For this review, use the dimensioned drawing (mm, ordinates from the lowest corner) and the shaded views. A direction names the side the tool comes from. Round coordinates to 2 decimals unless told otherwise and drop trailing zeros. Loops run counter-clockwise (first coordinate to the right, second up) from the corner with the lowest first, then second, coordinate; pieces in that order, holes last. Notation, with made-up numbers: M -13.5,58 L 13.5,58 A30 ccw 13.5,90 Z; hole C 58.25,15.5 d5. An arc over 180 degrees is marked long. One line per item, written item: value. Start each with the question number.
Item 1: For line 1 along Y through (x, z) = (32.25, 12.5); line 2 along Y through (x, z) = (32, 3); line 3 along Y through (x, z) = (31, 14.25), list the stretches that pass through material, from the lowest coordinate up.
Item 2: We need section A-A (x = 38). Write out the cut boundary in (y, z).
Item 3: We need section B-B (y = 50). Write out the cut boundary in (x, z).
Item 4: Clearance check with flat-ended pins moving along their axes: pin 1 (1.5 mm diameter, centred on x = 30, z = 10.5, fed in from -Y); pin 2 (2.5 mm diameter, centred on y = 48.5, z = 12, fed in from +X). State where each tip first meets the part, or that it passes through.
Item 5: We need section C-C (x = 22). Write out the cut boundary in (y, z), then the cut area to 3 significant figures.
Item 6: For the marked faces 5 and 6, list the 3-axis set-ups (+Z, -Z, +X, -X, +Y, -Y) from which the entire face can be reached by the end or side of a thin tool; tool diameter is ignored.
Item 7: We need section D-D (z = 12.5). Write out the cut boundary in (x, y), then the cut area to 3 significant figures.
Item 8: Mouldability with a two-part tool opening along Z and no side actions: class the marked faces 1, 2, 3 and 4 as released by +Z, released by -Z, zero draft, split by the parting line, or undercut.
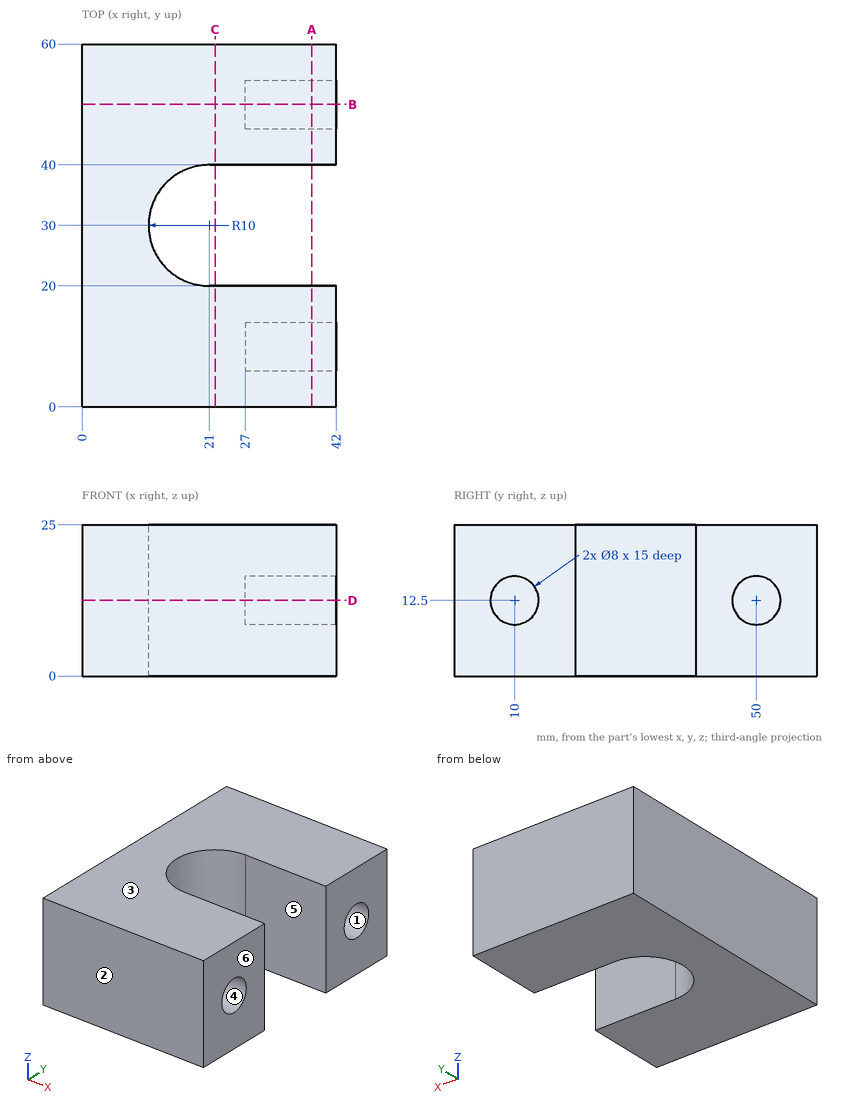
A:
1. line 1: 0 to 6, 14 to 20, 40 to 46, 54 to 60
1. line 2: 0 to 20, 40 to 60
1. line 3: 0 to 6.4, 13.6 to 20, 40 to 46.4, 53.6 to 60
2. outline: M 0,0 L 20,0 L 20,25 L 0,25 Z; M 40,0 L 60,0 L 60,25 L 40,25 Z; hole C 10,12.5 d8; hole C 50,12.5 d8
3. outline: M 0,0 L 42,0 L 42,8.5 L 27,8.5 L 27,16.5 L 42,16.5 L 42,25 L 0,25 Z
4. pin 1: y = 0
4. pin 2: x = 27
5. outline: M 0,0 L 20,0 L 20,25 L 0,25 Z; M 40,0 L 60,0 L 60,25 L 40,25 Z
5. area: 1,000 mm2
6. face 5: +Z, -Z, +X
6. face 6: +Z, -Z, +X, +Y, -Y
7. outline: M 0,0 L 42,0 L 42,6 L 27,6 L 27,14 L 42,14 L 42,20 L 21,20 A10 cw 21,40 L 42,40 L 42,46 L 27,46 L 27,54 L 42,54 L 42,60 L 0,60 Z
7. area: 1,700 mm2
8. face 1: undercut
8. face 2: zero draft
8. face 3: released by +Z
8. face 4: undercut
